Verification items for the finished model (mm, model axes). Coordinates: 2 decimals unless noted, no trailing zeros. Loops run counter-clockwise (first coordinate to the right, second up) from the corner with the lowest first, then second, coordinate; pieces in that order, holes last.
Q1. Mould release check, pull along Y, two halves, no side actions. Record for faces 1 (the face through (17, 92, -114)), 2 (the face through (12, 2755, -200)), 3 (the face through (8, 67, -114)): +Y half, -Y half, draft (parallel to the pull), parting line (faces both ways), or undercut.
Q2. Sectioned sample at B-B (z = -122.5). Enter the section's corners in (x, y), then the cut area to 3 significant figures.
Q3. Sectioned sample at C-C (z = 62). Count the separate pieces of the cut face and the enclosed holes in it, then the cut area to 3 significant figures.
Q4. Material ranges on probe 1 along Y at (x, z) = (22, -113); probe 2 along Z at (x, y) = (13.5, 178.5); probe 3 along Z at (x, y) = (22, 572.5), recorded low to high.
Q5. Sectioned sample at A-A (x = -22). Enter the section's corners in (y, z).
Q6. Go/stop test with flat-tipped pins: P1, Ø6, axis at x = 24.5, y = 2191, coming from the -Z side; P2, Ø2, axis at x = 12.5, z = 27, coming from the +Y side; P3, Ø12.5, axis at x = 40, y = 1480, coming from the +Z side. Record where each tip stops, or that it passes through.
Q7. Sectioned sample at D-D (y = 2192). Enter the section's corners in (x, z), then the cut area to 3 significant figures.
Autodesk Inventor part; units mm, degrees
ref_plane "YZ Plane" through (0, 0, 0) normal (1, 0, 0) x (0, 1, 0)
ref_plane "XZ Plane" through (0, 0, 0) normal (0, 1, 0) x (-1, 0, 0)
ref_plane "XY Plane" through (0, 0, 0) normal (0, 0, 1) x (1, 0, 0)
sketch "Sketch1" plane through (0, 0, 0) normal (0, 0, 1) x (1, 0, 0)
  line L0 (0, 0) -> (25, 0)
  line L1 (25, 0) -> (25, 2900)
  line L2 (25, 2900) -> (0, 2900)
  line L3 (0, 2900) -> (0, 0)
  dimension "d0" = 25
  dimension "d1" = 2900
extrude "Extrusion1" add sketch "Sketch1" along normal blind 25
sketch "Sketch2" plane through (0, 0, 0) normal (0, 0, -1) x (-1, 0, 0)
  line L0 (-25, 0) -> (-25, 2900)
  line L1 (0, 2900) -> (0, 0)
  line L2 (-25, 2900) -> (0, 2900)
  line L3 (0, 2900) -> (0, 2875)
  line L4 (0, 2875) -> (-25, 2875)
  line L5 (-25, 2875) -> (-25, 2900)
  dimension "d4" = 25
extrude "Extrusion2" add sketch "Sketch2" along normal blind 200
sketch "Sketch3" plane through (0, 2875, 0) normal (0, -1, 0) x (1, 0, 0)
  line L0 (0, -200) -> (0, 25)
  line L1 (25, -200) -> (25, 25)
  line L2 (0, -200) -> (25, -200)
  line L3 (25, -200) -> (25, -175)
  line L4 (25, -175) -> (0, -175)
  line L5 (0, -175) -> (0, -200)
  point P0 (0, 0)
  dimension "d7" = 25
extrude "Extrusion3" add sketch "Sketch3" along normal blind 200
sketch "Sketch4" plane through (0, 2875, -175) normal (0, 0, 1) x (1, 0, 0)
  line L0 (25, -200) -> (0, -200)
  line L1 (25, 25) -> (25, -200)
  line L2 (0, -200) -> (25, -200)
  line L3 (25, -200) -> (25, -175)
  line L4 (25, -175) -> (0, -175)
  line L5 (0, -175) -> (0, -200)
  point P0 (0, -2875)
  dimension "d10" = 25
extrude "Extrusion4" add sketch "Sketch4" along normal up to next
sketch "Sketch6" plane through (0, 0, 25) normal (-1, 0, 0) x (0, 0, 1)
  line L0 (-225, 2900) -> (-225, 2675)
  line L1 (-225, 2675) -> (-220, 2675)
  line L2 (-220, 2675) -> (-220, 2700)
  line L3 (-220, 2700) -> (-225, 2700)
  line L4 (-225, 2700) -> (-225, 2675)
  point P0 (-25, 0)
  dimension "d13" = 5
  dimension "d14" = 25
extrude "Extrusion5" add sketch "Sketch6" along normal blind 50 and the other way blind 75
pattern_linear "Rectangular Pattern1" count 3 spacing 1404 along (0, -1, 0) of "Extrusion2"
sketch "Sketch7" plane through (0, 0, 25) normal (-1, 0, 0) x (0, 0, 1)
  line L0 (-225, 1496) -> (-225, 1471)
  line L1 (-25, 1471) -> (-225, 1471)
  line L2 (-225, 1496) -> (-220, 1496)
  line L3 (-220, 1496) -> (-220, 1471)
  line L4 (-220, 1471) -> (-225, 1471)
  line L5 (-225, 1471) -> (-225, 1496)
  point P0 (-25, 0)
  dimension "d22" = 5
extrude "Extrusion6" add sketch "Sketch7" along normal blind 50 and the other way blind 75
pattern_linear "Rectangular Pattern2" count 2 spacing 1404 along (0, -1, 0) of "Extrusion6"
sketch "Sketch8" plane through (0, 0, 25) normal (-1, 0, 0) x (0, 0, 1)
  arc A0 (-0.0707, 2610) -> (83.9293, 2610) centre (41.9293, 2610) ccw
  arc A1 (3.9293, 2610) -> (79.9293, 2610) centre (41.9293, 2610) ccw
  line L0 (-0.0707, 2610) -> (3.9293, 2610)
  line L1 (0, 0) -> (0, 2900)
  line L2 (79.9293, 2610) -> (83.9293, 2610)
  line L3 (0, 2900) -> (0, 0)
  line L4 (0, 2900) -> (42, 2900)
  point P0 (-25, 0)
  dimension "d31" = 4
  dimension "d39" = 42
  dimension "d40" = 290
extrude "Extrusion7" add sketch "Sketch8" against normal up to surface (25 mm away)
pattern_linear "Rectangular Pattern3" count 8 spacing 338 along (0, -1, 0) of "Extrusion7"
sketch "Sketch10" plane through (0, 2900, -200) normal (-1, 0, 0) x (0, 0, 1)
  line L0 (200, -2900) -> (225, -2900)
  line L1 (225, -2900) -> (267, -2900)
  dimension "d41" = 42
properties part number "Stand"
Geometry check:
1. face 1: undercut
1. face 2: draft
1. face 3: -Y half
2. outline: (0, 67) - (25, 67) - (25, 92) - (0, 92) - close; (0, 1471) - (25, 1471) - (25, 1496) - (0, 1496) - close; (0, 2675) - (25, 2675) - (25, 2700) - (0, 2700) - close; (0, 2875) - (25, 2875) - (25, 2900) - (0, 2900) - close
2. area: 2,500 mm2
3. separate pieces: 8
3. enclosed holes: 0
3. area: 806 mm2
4. probe 1: y = 67 to 92, 1471 to 1496, 2675 to 2700, 2875 to 2900
4. probe 2: z = 0 to 25
4. probe 3: z = 0 to 25, 26.02 to 30.14, 103.72 to 107.84
5. outline: (67, -200) - (92, -200) - (92, -195) - (67, -195) - close; (1471, -200) - (1496, -200) - (1496, -195) - (1471, -195) - close; (2675, -200) - (2700, -200) - (2700, -195) - (2675, -195) - close
6. P1: stops at z = 0
6. P2: stops at y = 2610
6. P3: stops at z = -195
7. outline: (0, 0) - (25, 0) - (25, 25) - (0, 25) - close
7. area: 625 mm2
